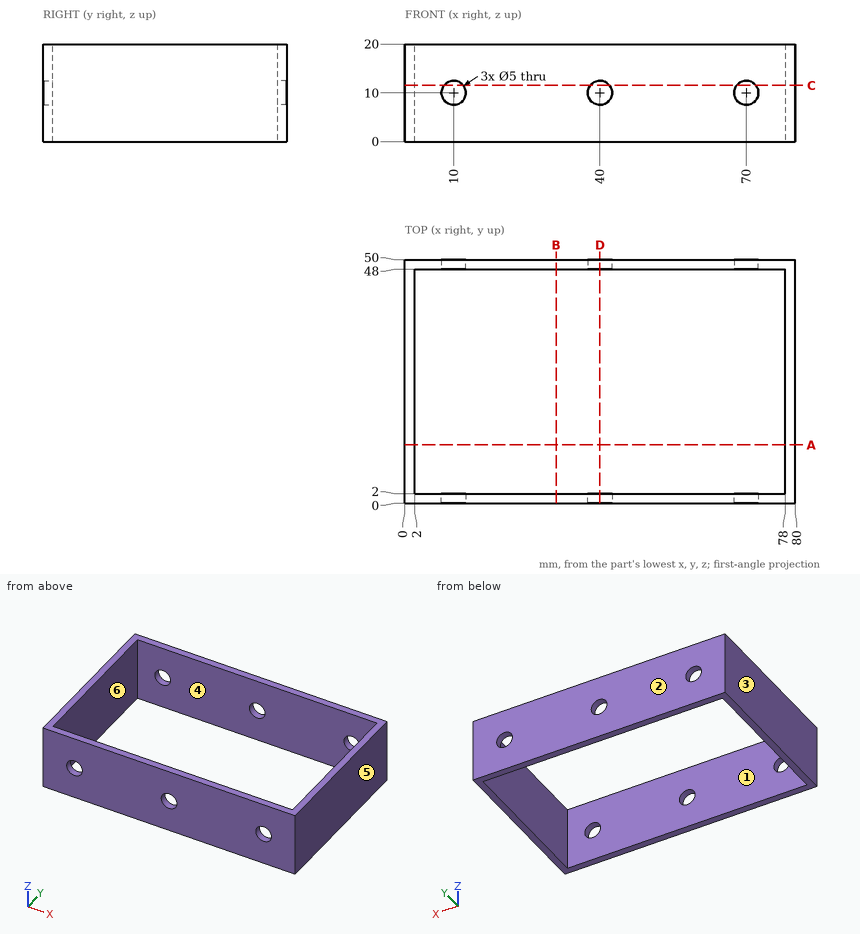
Here's the drawing with two shaded views (mm, measured from the low corner). I have some questions. A direction names the side the tool comes from. Give positions to 0.01 mm unless a question says otherwise; leave off trailing zeros. Write each loop counter-clockwise with the first axis right and the second up, starting at its lowest first coordinate (ties: lowest second). Pieces come first, ordered by that corner, then holes. Notation, with made-up numbers: (49, 26.5) -> (104, 26.5) arc R35 ccw to (104, 58.5) -> close; hole circle Ø9 at (-36, 54). An arc over 180 degrees is marked (long way). Answer as a JSON object with one key per item and string values. Group by question number.
Item 1: I'm going to push a flat-ended pin straight in: P1, Ø10, axis at y = 35.5, z = 10.5, coming from the -X side. Where does the tip first touch, or does it pass through?
Item 2: Suppose I cut it at C-C (z = 11.5). State how many separate pieces and enclosed holes the cut face has, plus the area to 3 significant figures.
Item 3: Please list where these lines run through material, in increasing order: line 1 (X direction, y = 1.45, z = 10); line 2 (Y direction, x = 60, z = 1.5); line 3 (X direction, y = 16.5, z = 5.25). Write a range as [from, to].
Item 4: We'd pull the mould along Y, two halves only. Please class the marked faces 1, 2, 3 and 4: +Y half, -Y half, draft (parallel to the pull), parting line (faces both ways), or undercut.
Item 5: Suppose I cut it at D-D (x = 40). Please give me the cut outline in (y, z).
Item 6: For the marked faces 5 and 6, which set-ups out of +Z, -Z, +X, -X, +Y, -Y let a thin tool reach every point of the face, with its end or its side?
Item 7: Suppose I cut it at A-A (y = 12). Please give me the cut outline in (x, z), plus the area to 3 significant figures.
Item 8: Suppose I cut it at B-B (x = 31). Please give me the cut outline in (y, z).
Findings:
{
 "1": {"P1": "stops at x = 0"},
 "2": {"separate pieces": "6", "enclosed holes": "0", "area": "456 mm²"},
 "3": {"line 1": "x = [0, 7.5], [12.5, 37.5], [42.5, 67.5], [72.5, 80]", "line 2": "y = [0, 2], [48, 50]", "line 3": "x = [0, 2], [78, 80]"},
 "4": {"face 1": "undercut", "face 2": "+Y half", "face 3": "draft", "face 4": "undercut"},
 "5": {"outline": "(0, 0) -> (2, 0) -> (2, 7.5) -> (0, 7.5) -> close; (0, 12.5) -> (2, 12.5) -> (2, 20) -> (0, 20) -> close; (48, 0) -> (50, 0) -> (50, 7.5) -> (48, 7.5) -> close; (48, 12.5) -> (50, 12.5) -> (50, 20) -> (48, 20) -> close"},
 "6": {"face 5": "+Z, -Z, +X, +Y, -Y", "face 6": "+Z, -Z"},
 "7": {"outline": "(0, 0) -> (2, 0) -> (2, 20) -> (0, 20) -> close; (78, 0) -> (80, 0) -> (80, 20) -> (78, 20) -> close", "area": "80.0 mm²"},
 "8": {"outline": "(0, 0) -> (2, 0) -> (2, 20) -> (0, 20) -> close; (48, 0) -> (50, 0) -> (50, 20) -> (48, 20) -> close"}
}
